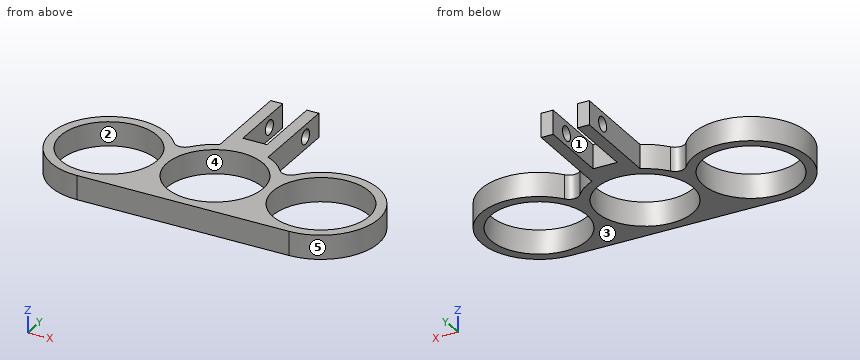
Autodesk Inventor part; units mm, degrees
ref_plane "YZ Plane" through (0, 0, 0) normal (1, 0, 0) x (0, 1, 0)
ref_plane "XZ Plane" through (0, 0, 0) normal (0, 1, 0) x (-1, 0, 0)
ref_plane "XY Plane" through (0, 0, 0) normal (0, 0, 1) x (1, 0, 0)
sketch "Sketch1" plane through (0, 0, 0) normal (0, 0, 1) x (1, 0, 0)
  line L0 (-2.5, 10) -> (-2.5, 20)
  line L1 (2.5, 10) -> (2.5, 25)
  line L2 (2.5, 25) -> (5, 25)
  arc A0 (6.0006, 0.0769) -> (6, -0.0245) centre (14, -0.0245) ccw
  line L3 (-2.5, 10) -> (2.5, 10)
  line L4 (-5, 20) -> (-5, 5.9087)
  line L5 (0, 10) -> (0, 17.0552) construction
  line L6 (5, 25) -> (5, 5.9087)
  circle A1 centre (0, -5) radius 10
  line L7 (0, -5) -> (-38, -5) construction
  arc A2 (-5, 5.9087) -> (-9.4286, 2.4231) centre (0, -5) ccw
  arc A3 (12, -5) -> (22, -15) centre (22, -5) ccw
  arc A4 (9.4286, 2.4231) -> (5, 5.9087) centre (0, -5) ccw
  line L8 (0, -17) -> (22, -17)
  circle A5 centre (-22, -5) radius 10
  arc A6 (-12.5714, 2.4231) -> (-22, -17) centre (-22, -5) ccw
  arc A7 (-12.5714, 2.4231) -> (-9.4286, 2.4231) centre (-11, 3.6603) ccw
  line L9 (-22, -17) -> (0, -17)
  circle A8 centre (22, -5) radius 10
  arc A9 (22, -17) -> (12.5714, 2.4231) centre (22, -5) ccw
  arc A10 (9.4286, 2.4231) -> (12.5714, 2.4231) centre (11, 3.6603) ccw
  line L10 (-2.5, 20) -> (-2.5, 25)
  line L11 (-2.5, 25) -> (-5, 25)
  line L12 (-5, 25) -> (-5, 20)
  point P0 (0, 0)
  point P1 (8, 0)
  point P2 (-32, -5)
  point P3 (-12, -5)
  point P4 (-34, -5)
  point P5 (32, -5)
  point P6 (11, -9.7958)
  point P7 (-5, -15.9087)
  point P8 (38, -5)
  point P9 (32, -5)
  point P10 (34, -5)
  dimension "d12" = 2.5
  dimension "d13" = 10
  dimension "d14" = 2.5
  dimension "d15" = 15
  dimension "d24" = 20
  dimension "d36" = 2
  dimension "d44" = 5
extrude "Extrusion1" add sketch "Sketch1" along normal blind 5
sketch "Sketch3" plane through (0, 0, 5) normal (0, 0, 1) x (1, 0, 0)
  circle A0 centre (0, -5) radius 10
  point P0 (0, 0)
  dimension "d26" = 20
extrude "Extrusion3" cut sketch "Sketch3" against normal blind 5
fillet "Fillet2" [suppressed]
sketch "Sketch4" plane through (5, 5.9087, 0) normal (1, 0, 0) x (0, 0, -1)
  line L0 (0, 19.0913) -> (-5, 19.0913) construction
  line L1 (-2.5, 19.0913) -> (-2.5, 14.0913) construction
  circle A0 centre (-2.5, 14.0913) radius 1.5
  point P0 (0, -5.9087)
  dimension "d30" = 5
  dimension "d31" = 3
extrude "Extrusion4" cut sketch "Sketch4" against normal blind 10
properties part number "beta_dummy"
Could you check a few things on this model? Use its own coordinates, in mm. Face numbers are marked on the shaded views. A direction names the side the tool comes from. Give positions to 0.01 mm unless a question says otherwise; leave off trailing zeros. Order: outer loops, then holes, each group sorted by start corner. A loop starts at its lowest first (then second) coordinate and runs counter-clockwise, first axis right, second up.
Q1. For the marked faces 1 and 2, which set-ups out of +Z, -Z, +X, -X, +Y, -Y let a thin tool reach every point of the face, with its end or its side?
Q2. We'd pull the mould along X, two halves only. Please class the marked faces 3, 4 and 5: +X half, -X half, draft (parallel to the pull), parting line (faces both ways), or undercut.
Q3. Suppose I cut it at A-A, the plane z = 2.5. Write out the boundary of the cut face in (x, y).
Q4. Suppose I cut it at D-D, the plane y = 20. Write out the boundary of the cut face in (x, z).
Q5. If I drill on line 1 along X through (y, z) = (18.5, 0.3); line 2 along X through (y, z) = (1.5, 3.2); line 3 along Y through (x, z) = (-0.5, 2), over which ranges is the centre line in solid material (lowest first)?
Q6. Suppose I cut it at C-C, the plane y = -5. Write out the boundary of the cut face in (x, z).
Q7. I'm going to push flat-ended pins straight in: P1, Ø2.5, axis at y = 14, z = 1.5, coming from the -X side; P2, Ø2.5, axis at y = 17, z = 2, coming from the +X side. Where does each tip first touch, or does it pass through?
Q8. Suppose I cut it at B-B, the plane x = 0. Write out the boundary of the cut face in (y, z).
Solution:
1. face 1: +Z, -Z, +Y
1. face 2: +Z, -Z
2. face 3: draft
2. face 4: undercut
2. face 5: undercut
3. outline: (-22, -17) - (22, -17) arc R12 ccw (long way) to (12.57, 2.42) arc R2 cw to (9.43, 2.42) arc R12 ccw to (5, 5.91) - (5, 18.5) - (2.5, 18.5) - (2.5, 10) - (-2.5, 10) - (-2.5, 18.5) - (-5, 18.5) - (-5, 5.91) arc R12 ccw to (-9.43, 2.42) arc R2 cw to (-12.57, 2.42) arc R12 ccw (long way) to start; (-5, 21.5) - (-2.5, 21.5) - (-2.5, 25) - (-5, 25) - close; (2.5, 21.5) - (5, 21.5) - (5, 25) - (2.5, 25) - close; hole circle Ø20 at (-22, -5); hole circle Ø20 at (0, -5); hole circle Ø20 at (22, -5)
4. outline: (-5, 0) - (-2.5, 0) - (-2.5, 1) - (-5, 1) - close; (-5, 4) - (-2.5, 4) - (-2.5, 5) - (-5, 5) - close; (2.5, 0) - (5, 0) - (5, 1) - (2.5, 1) - close; (2.5, 4) - (5, 4) - (5, 5) - (2.5, 5) - close
5. line 1: x = -5 to -2.5, 2.5 to 5
5. line 2: x = -32.09 to -29.6, -14.4 to -7.6, 7.6 to 14.4, 29.6 to 32.09
5. line 3: y = -17 to -14.99, 4.99 to 10
6. outline: (-34, 0) - (-32, 0) - (-32, 5) - (-34, 5) - close; (-12, 0) - (-10, 0) - (-10, 5) - (-12, 5) - close; (10, 0) - (12, 0) - (12, 5) - (10, 5) - close; (32, 0) - (34, 0) - (34, 5) - (32, 5) - close
7. P1: stops at x = -5
7. P2: stops at x = 5
8. outline: (-17, 0) - (-15, 0) - (-15, 5) - (-17, 5) - close; (5, 0) - (10, 0) - (10, 5) - (5, 5) - close
